Can you work these out from the model? Positions are in its coordinate system, mm. Face numbers are marked on the shaded views. A direction names the side the tool comes from. Give positions to 0.01 mm unless a question says otherwise; leave off trailing zeros. Loops run counter-clockwise (first coordinate to the right, second up) from the corner with the lowest first, then second, coordinate; pieces in that order, holes last. Notation, with made-up numbers: (55.25, 49.5) -> (61.25, 49.5) arc R35 cw to (61.25, 84.5) -> close; hole circle Ø8 at (42, 76.25). An arc over 180 degrees is marked (long way). Return JSON: item names as keys, results as strings. Group by question number.
Q1. Suppose I cut it at A-A, the plane z = 0. Please give me the cut outline in (x, y), and give its area (3 significant figures).
Q2. Thinking about a two-plate mould opening in X: for the marked faces 3, 4 and 5, which applies, pulls with the +X half, pulls with the -X half, needs draft (parallel to the pull), parting line crosses it, or undercut?
Q3. Suppose I cut it at B-B, the plane y = 4. Please give me the cut outline in (x, z), and give its area (3 significant figures).
Q4. Which directions (+Z, -Z, +X, -X, +Y, -Y) give clear straight access to the entire face, cutting with the end or side of a thin tool? Please do the marked faces 1 and 2.
Q5. Will these pins go through, and if not, where does the flat tip stop? pin 1 (8 mm diameter, centred on x = 17, y = 8, fed in from -Z); pin 2 (11 mm diameter, centred on x = -11.5, z = -4, fed in from -Y).
Q6. Suppose I cut it at C-C, the plane x = 0. Please give me the cut outline in (y, z).
Q7. I need wall thicknesses on line 1 along X through (y, z) = (-8.5, 14.5); line 2 along Y through (x, z) = (30, 9); line 3 along X through (y, z) = (11.5, 7.5). Which ranges of each line are inside material? Lowest first, please. Write a range as [from, to].
Q8. Suppose I cut it at D-D, the plane z = -5. Please give me the cut outline in (x, y).
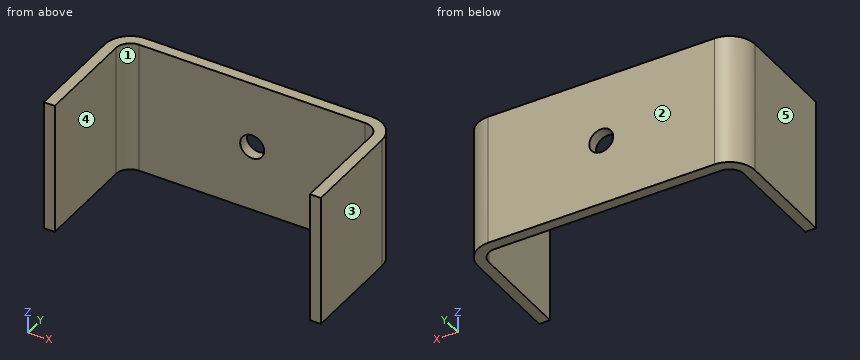
```python
from build123d import *

# Parameters (mm, degrees)
BASE_FLANGE1_DEPTH = 18.1
CUT_EXTRUDE1_REACH = 56.683
SKETCH6_R          = 3.3


# Sheet-metal steps are written as plain solids
with BuildPart() as part:
    # Sketch1 → Base-Flange1 (new, symmetric)
    with BuildSketch(Plane.XY):
        with BuildLine():
            Line((-38.1, -17.4), (-38.1, 10.4))
            ThreePointArc((-38.1, 10.4), (-36.049747468, 15.349747468), (-31.1, 17.4))
            Line((-31.1, 17.4), (31.1, 17.4))
            ThreePointArc((31.1, 17.4), (36.049747468, 15.349747468), (38.1, 10.4))
            Line((38.1, 10.4), (38.1, -17.4))
            Line((38.1, -17.4), (35.1, -17.4))
            Line((35.1, -17.4), (35.1, 10.4))
            ThreePointArc((35.1, 10.4), (33.928427125, 13.228427125), (31.1, 14.4))
            Line((31.1, 14.4), (-31.1, 14.4))
            ThreePointArc((-31.1, 14.4), (-33.928427125, 13.228427125), (-35.1, 10.4))
            Line((-35.1, 10.4), (-35.1, -17.4))
            Line((-35.1, -17.4), (-38.1, -17.4))
        make_face()
    extrude(amount=BASE_FLANGE1_DEPTH, both=True)

    # Sketch6 → Cut-Extrude1 (cut, up to next)
    with BuildSketch(Plane(origin=(0, 17.4, 0), x_dir=(1, 0, 0), z_dir=(0, 1, 0)), mode=Mode.PRIVATE) as cut_extrude1_sk1:
        with Locations(Location((0, 0, 0), (0, 0, 270))):
            Circle(SKETCH6_R)
    cut_extrude1_tool1 = extrude(cut_extrude1_sk1.sketch, amount=-CUT_EXTRUDE1_REACH, mode=Mode.PRIVATE) & part.part
    add(cut_extrude1_tool1.solids().sort_by_distance((0, 17.4, 0))[0], mode=Mode.SUBTRACT)


solid = part.part
```
Ans:
{
 "1": {"outline": "(-38.1, -17.4) -> (-35.1, -17.4) -> (-35.1, 10.4) arc R4 cw to (-31.1, 14.4) -> (-3.3, 14.4) -> (-3.3, 17.4) -> (-31.1, 17.4) arc R7 ccw to (-38.1, 10.4) -> close; (3.3, 14.4) -> (31.1, 14.4) arc R4 cw to (35.1, 10.4) -> (35.1, -17.4) -> (38.1, -17.4) -> (38.1, 10.4) arc R7 ccw to (31.1, 17.4) -> (3.3, 17.4) -> close", "area": "385 mm^2"},
 "2": {"face 3": "pulls with the +X half", "face 4": "undercut", "face 5": "pulls with the -X half"},
 "3": {"outline": "(-38.1, -18.1) -> (-35.1, -18.1) -> (-35.1, 18.1) -> (-38.1, 18.1) -> close; (35.1, -18.1) -> (38.1, -18.1) -> (38.1, 18.1) -> (35.1, 18.1) -> close", "area": "217 mm^2"},
 "4": {"face 1": "+Z, -Z, -Y", "face 2": "+Z, -Z, +X, -X, +Y"},
 "5": {"pin 1": "passes through", "pin 2": "stops at y = 14.4"},
 "6": {"outline": "(14.4, -18.1) -> (17.4, -18.1) -> (17.4, -3.3) -> (14.4, -3.3) -> close; (14.4, 3.3) -> (17.4, 3.3) -> (17.4, 18.1) -> (14.4, 18.1) -> close"},
 "7": {"line 1": "x = [-38.1, -35.1], [35.1, 38.1]", "line 2": "y = [14.4, 17.4]", "line 3": "x = [-38.01, -34.95], [34.95, 38.01]"},
 "8": {"outline": "(-38.1, -17.4) -> (-35.1, -17.4) -> (-35.1, 10.4) arc R4 cw to (-31.1, 14.4) -> (31.1, 14.4) arc R4 cw to (35.1, 10.4) -> (35.1, -17.4) -> (38.1, -17.4) -> (38.1, 10.4) arc R7 ccw to (31.1, 17.4) -> (-31.1, 17.4) arc R7 ccw to (-38.1, 10.4) -> close"}
}
